from build123d import *

# Parameters (mm, degrees)
MODEL_R           = 1.4
MODEL_R_2         = 1
BRIDA_BASE1_DEPTH = 1


# Sheet-metal steps are written as plain solids
with BuildPart() as part:
    # Model → Brida base1 (new body)
    with BuildSketch(Plane.XY):
        with BuildLine():
            Line((40, 21.38389001), (40.2059904, -15.761563617))
            ThreePointArc((40.2059904, -15.761563617), (45.205990408, -20.761561608), (50.205990416, -15.761563617))
            Line((50.205990416, -15.761563617), (50.205990416, 21.38389001))
            ThreePointArc((50.205990416, 21.38389001), (59.282249533, 23.973347274), (61.871706797, 14.897088157))
            ThreePointArc((61.871706797, 14.897088157), (66.397009574, 27.571280603), (59.516453931, 39.13724245))
            ThreePointArc((59.516453931, 39.13724245), (57.297457404, 31.686860899), (49.524022567, 31.763291841))
            Line((49.524022567, 31.763291841), (49.524022567, 34.243690175))
            Line((49.524022567, 34.243690175), (40.681967849, 34.243690175))
            Line((40.681967849, 34.243690175), (40.681967849, 31.763291841))
            ThreePointArc((40.681967849, 31.763291841), (32.908533012, 31.686860899), (30.689536484, 39.13724245))
            ThreePointArc((30.689536484, 39.13724245), (23.808980842, 27.571280603), (28.334283619, 14.897088157))
            ThreePointArc((28.334283619, 14.897088157), (30.923740883, 23.973347274), (40, 21.38389001))
        make_face()
        with Locations((45.205990408, -15.7615616)):
            Circle(MODEL_R, mode=Mode.SUBTRACT)
        with Locations((45.205990408, -3.2615616)):
            Circle(MODEL_R_2, mode=Mode.SUBTRACT)
    extrude(amount=-BRIDA_BASE1_DEPTH)


solid = part.part
Work out the finished part from the listing and answer in its coordinate system (mm). Give positions to 0.01 mm unless a question says otherwise; leave off trailing zeros. Loops run counter-clockwise (first coordinate to the right, second up) from the corner with the lowest first, then second, coordinate; pieces in that order, holes last. Notation, with made-up numbers: (5.25, 71.25) -> (11.25, 71.25) arc R16 cw to (11.25, 81.25) -> close; hole circle Ø5 at (21.25, -28.75). An arc over 180 degrees is marked (long way). Use a Markdown table: item, result. Add a question column.
1) Consider line 1 along X through (y, z) = (27.5, -0.8); line 2 along Y through (x, z) = (26, -0.65); line 3 along Y through (x, z) = (29, -0.45). Determine where each line is inside the solid, lowest interval first.
2) The part is cut by section A-A, the plane z = -0.2. Determine the outline of the cut face in (x, y) (3 decimals), plus the area to 3 significant figures.
3) The part is cut by section B-B, the plane y = 14. Determine the outline of the cut face in (x, z).
4) Each of these flat-tipped pins is pushed along its axis until it touches: P1, Ø2.5, axis at x = 45.21, y = -15.76, coming from the -Z side; P2, Ø12, axis at x = 49.5, y = 9, coming from the +Z side. Where does it stop, or does it pass through?
5) For a pull along X with two mould halves and no side action, classify faces 1 (the cylindrical face through (66.415, 27.377, -0.493)), 2 (the cylindrical face through (44.207, -3.218, -0.493)), 3 (the flat face through (45, 14, -1)) as +X half, -X half, draft (parallel to the pull), parting line (faces both ways), or undercut.
6) The part is cut by section C-C, the plane x = 43. Determine the outline of the cut face in (y, z).
Reported:
| question | item | result |
|---|---|---|
| 1 | line 1 | x = 23.8 to 66.4 |
| 1 | line 2 | y = 17.89 to 34.2 |
| 1 | line 3 | y = 22.36 to 37.82 |
| 2 | outline | (28.334, 14.897) arc R6.674 cw to (40, 21.384) -> (40.206, -15.762) arc R5 ccw to (50.206, -15.762) -> (50.206, 21.384) arc R6.674 cw to (61.872, 14.897) arc R15.805 ccw to (59.516, 39.137) arc R6.46 cw to (49.524, 31.763) -> (49.524, 34.244) -> (40.682, 34.244) -> (40.682, 31.763) arc R6.46 cw to (30.69, 39.137) arc R15.805 ccw to start; hole circle Ø2.8 at (45.206, -15.762); hole circle Ø2 at (45.206, -3.262) |
| 2 | area | 871 mm^2 |
| 3 | outline | (40.04, -1) -> (50.21, -1) -> (50.21, 0) -> (40.04, 0) -> close |
| 4 | P1 | passes through |
| 4 | P2 | stops at z = 0 |
| 5 | face 1 | +X half |
| 5 | face 2 | undercut |
| 5 | face 3 | draft |
| 6 | outline | (-20.25, -1) -> (34.24, -1) -> (34.24, 0) -> (-20.25, 0) -> close |
